from build123d import *

# Parameters (mm, degrees)
F2_R     = 1
F3_SIZE  = 1
F5_DEPTH = 2.88


# Not quite as in the source:
# - a fillet or chamfer that OpenCascade refuses, or shapes differently, is made with other operations: its cross-section is extruded or revolved along the edge and cut away or added


with BuildPart() as f1:
    # F0 (on Front) → F1 (revolve)
    with BuildSketch(Plane.XZ):
        Polygon((-4, 0), (0, 0), (0, 31.056624327), (-2.5, 32.5), (-2.5, 38), (-6.5, 38), (-6.5, 30), (-4, 30), (-4, 26.25), (-3.5, 26), (-4, 25.75), align=None)
    revolve(axis=Axis((0, 0, 18.332445994), (0, 0, 1)))

    # F2
    f2_edges = [f1.edges().sort_by_distance(p)[0] for p in [
        (6.5, 0, 38),
    ]]
    fillet(f2_edges, radius=F2_R)

    # F3
    f3_edges = [f1.edges().sort_by_distance(p)[0] for p in [
        (4, 0, 0),
    ]]
    chamfer(f3_edges, length=F3_SIZE)

    # F4 (on face) → F5 (cut)
    with BuildSketch(Plane.XY.offset(38)):
        Polygon((-1.7320508076, -3), (1.7320508076, -3), (3.4641016151, 0), (1.7320508076, 3), (-1.7320508076, 3), (-3.4641016151, 0), align=None)
    extrude(amount=-F5_DEPTH, mode=Mode.SUBTRACT)

    # F6: chamfer of 1.5 x 2.5980762114 on 1 edges, made by hand


with BuildPart() as f6_tool2:
    # F6_s3 → F6_t4 (revolve)
    with BuildSketch(Plane.XZ):
        Polygon((-5.0980762114, 35.12), (-2.5, 33.62), (-2.5, 35.12), align=None)
    revolve(axis=Axis((0, 0, 35.12), (0, 0, 1)))

    split(bisect_by=Plane(origin=(-2.5980762114, -1.5, 0), x_dir=(0, 0, 1), z_dir=(0.8660254038, 0.5, 0)), keep=Keep.TOP)

    split(bisect_by=Plane(origin=(-2.5980762114, 1.5, 0), x_dir=(0, 0, 1), z_dir=(0.8660254038, -0.5, 0)), keep=Keep.TOP)

    split(bisect_by=Plane.XZ.offset(-3), keep=Keep.TOP)

    split(bisect_by=Plane(origin=(2.5980762114, 1.5, 0), x_dir=(0, 0, 1), z_dir=(-0.8660254038, -0.5, 0)), keep=Keep.TOP)

    split(bisect_by=Plane(origin=(2.5980762114, -1.5, 0), x_dir=(0, 0, 1), z_dir=(-0.8660254038, 0.5, 0)), keep=Keep.TOP)

    split(bisect_by=Plane.XZ.offset(3), keep=Keep.BOTTOM)


with BuildPart() as f1_1:
    add(f1.part)

    # F6_t1: cut F6_tool2
    add(f6_tool2.part, mode=Mode.SUBTRACT)


solid = f1_1.part
The listing builds one solid part. Answer for the finished solid, in the listing's coordinates (mm). A direction names the side the tool comes from. Coordinates: 2 decimals unless noted, no trailing zeros. Write each loop counter-clockwise with the first axis right and the second up, starting at its lowest first coordinate (ties: lowest second). Pieces come first, ordered by that corner, then holes. Notation, with made-up numbers: (77.5, 62.5) - (85.5, 62.5) arc R23 cw to (85.5, 80.5) - close; hole circle Ø11 at (-32.5, -38.5). An arc over 180 degrees is marked (long way). Put each result on its own line as item: value.
1. Determine the mould class of faces 1 (the face through (0.867, 3.905, 13.202)), 2 (the face through (0, 3, 36)), 3 (the face through (-3, -3, 30)) for opening direction Y: pulls with the +Y half, pulls with the -Y half, needs draft (parallel to the pull), parting line crosses it, or undercut.
Answer sheet:
face 1: parting line crosses it
face 2: undercut
face 3: needs draft
2. Find the intervals of material crossed by line 1 along Y through (x, z) = (0, 33); line 2 along Z through (x, y) = (-4.75, -2), in increasing order. Write a range as from..to.
Answer sheet:
line 1: y = -6.5..-2.5, 2.5..6.5
line 2: z = 30..38
3. The part is cut by section A-A on z = 36. Give the vertices of the cut face in (x, y), plus the area to 3 significant figures.
Answer sheet:
outline: circle Ø13 at (0, 0); hole (-3.46, 0) - (-1.73, -3) - (1.73, -3) - (3.46, 0) - (1.73, 3) - (-1.73, 3) - close
area: 102 mm^2
4. The part is cut by section B-B on z = 24.5. Give the vertices of the cut face in (x, y).
Answer sheet:
outline: circle Ø8 at (0, 0)
5. A tool of negligible diameter and unlimited length cuts with its end or side. For faces 4 (the face through (0.867, 3.905, 28.099)), 5 (the face through (0, -3, 36)), 6 (the face through (5.158, 3.955, 33.451)), from which of +Z, -Z, +X, -X, +Y, -Y can it reach the whole face along a straight path? Write none if from no direction.
Answer sheet:
face 4: -Z
face 5: +Z
face 6: +Z, -Z
6. Flat-ended cylindrical pins translate along their axes: pin 1 Ø1.7 at (x, z) = (-1, 35) entering from +Y; pin 2 Ø1.5 at (y, z) = (-2.5, 6) entering from +X; pin 3 Ø1.7 at (x, z) = (1, 36) entering from -Y. Find the tip coordinate at first contact, or state that the pin passes through.
Answer sheet:
pin 1: stops at y = 6.5
pin 2: stops at x = 3.6
pin 3: stops at y = -6.5
